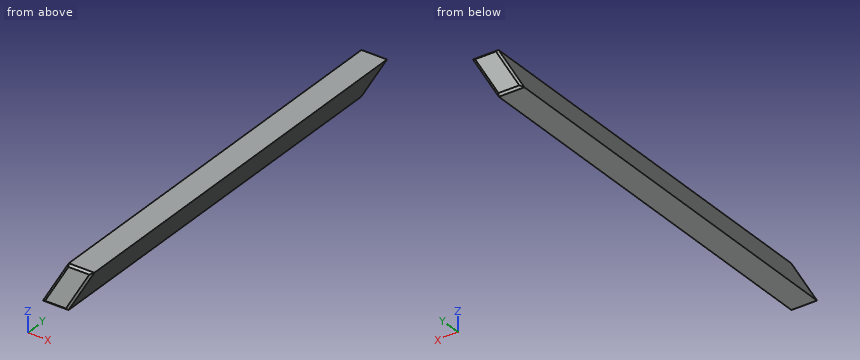
```python
from build123d import *

# Parameters (mm, degrees)
F1_DEPTH = 100
F2_SIZE  = 0.5


with BuildPart() as f1:
    # F0 (on Front) → F1 (new body)
    with BuildSketch(Plane.XZ):
        Polygon((6.235383, 10.8), (0, 0), (6.177648, 0), (12.413031, 10.8), align=None)
    extrude(amount=F1_DEPTH)

    # F2
    f2_edges = [f1.edges().sort_by_distance(p)[0] for p in [
        (9.324207, -100, 10.8),
        (3.117691, -100, 5.4),
        (9.295339, -100, 5.4),
        (3.088824, -100, 0),
        (9.295339, 0, 5.4),
        (3.117691, 0, 5.4),
        (3.088824, 0, 0),
        (9.324207, 0, 10.8),
    ]]
    chamfer(f2_edges, length=F2_SIZE)


solid = f1.part
```
The listing builds one solid part. Answer for the finished solid, in the listing's coordinates (mm). Give positions to 0.01 mm unless a question says otherwise; leave off trailing zeros. Write each loop counter-clockwise with the first axis right and the second up, starting at its lowest first coordinate (ties: lowest second). Pieces come first, ordered by that corner, then holes. Notation, with made-up numbers: (2, 57) - (17, 57) arc R8 cw to (17, 66) - close; hole circle Ø10 at (53.5, 22). An arc over 180 degrees is marked (long way). Use one line per item in the form item = value. Start each with the question number.
1) Flat-ended cylindrical pins translate along their axes: pin 1 Ø1 at (x, y) = (4.5, -37.5) entering from +Z; pin 2 Ø2 at (x, y) = (2, -63.5) entering from +Z; pin 3 Ø1 at (x, y) = (3, -11.5) entering from +Z. Find the tip coordinate at first contact, or state that the pin passes through.
2) Find section C-C on y = -20.5. Determine the outline of the cut face in (x, z), plus the area to 3 significant figures.
3) Consider line 1 along X through (y, z) = (-75, 10); line 2 along Z through (x, y) = (8, -82); line 3 along X through (y, z) = (-49, 5). Determine where each line is inside the solid, lowest interval first. Write a range as from..to.
4) Find section A-A on x = 3.5. Determine the outline of the cut face in (y, z), plus the area to 3 significant figures.
5) Find section B-B on z = 9. Determine the outline of the cut face in (x, y).
Geometry results:
q1.pin_1 = 8.66
q1.pin_2 = 5.2
q1.pin_3 = 6.06
q2.outline = (0, 0) - (6.18, 0) - (12.41, 10.8) - (6.24, 10.8) - close
q2.area = 66.7 mm2
q3.line_1 = 5.77..11.95
q3.line_2 = 3.16..10.8
q3.line_3 = 2.89..9.06
q4.outline = (-100, 0.5) - (-99.5, 0) - (-0.5, 0) - (0, 0.5) - (0, 5.06) - (-0.5, 6.06) - (-99.5, 6.06) - (-100, 5.06) - close
q4.area = 605 mm2
q5.outline = (5.2, -99.5) - (5.77, -100) - (10.8, -100) - (11.37, -99.5) - (11.37, -0.5) - (10.8, 0) - (5.77, 0) - (5.2, -0.5) - close
